```python
from build123d import *

# Parameters (mm, degrees)
F0_W     = 75.8
F0_H     = 10
F1_DEPTH = 2
F2_R     = 1
F4_D     = 3.5


with BuildPart() as f1:
    # F0 (on Front) → F1 (new body)
    with BuildSketch(Plane.XZ):
        Rectangle(F0_W, F0_H)
    extrude(amount=F1_DEPTH)

    # F2
    f2_edges = [f1.edges().sort_by_distance(p)[0] for p in [
        (-37.9, -1, 5),
        (37.9, -1, 5),
    ]]
    fillet(f2_edges, radius=F2_R)

    # F4 (through all)
    with Locations(Plane.XZ.offset(2)):
        with Locations((30, -0.5), (-30, -0.5)):
            Hole(F4_D / 2)


solid = f1.part
```
Verification items for the finished model (mm, model axes). Give positions to 0.01 mm unless a question says otherwise; leave off trailing zeros. Order: outer loops, then holes, each group sorted by start corner. A loop starts at its lowest first (then second) coordinate and runs counter-clockwise, first axis right, second up. Notation, with made-up numbers: M 16,-4 L 35,-4 A9 cw 35,1 Z; hole C 52.25,2 d8. An arc over 180 degrees is marked long. Answer in a Markdown table with one row per item. Add a question column.
Item 1: Section check B-B, the plane x = 30. Enter the section's corners in (y, z), and give its area (3 significant figures).
Item 2: Section check A-A, the plane z = -0.5. Enter the section's corners in (x, y), and give its area (3 significant figures).
Item 3: Scan lines: probe 1 along Z at (x, y) = (30, -0.85); probe 2 along X at (y, z) = (-0.9, 0.5); probe 3 along X at (y, z) = (-0.75, -1.75). Record each from-to range of solid material in increasing order. Write a range as from..to.
Item 4: Mould release check, pull along Z, two halves, no side actions. Record for faces 1 (the flat face through (-1, -1, -5)), 2 (the flat face through (-1, 0, 0)), 3 (the cylindrical face through (31.75, -0.99, -0.42)): released by +Z, released by -Z, zero draft, split by the parting line, or undercut.
Item 5: Section check C-C, the plane y = -1.3. Enter the section's corners in (x, z), and give its area (3 significant figures).
Filled sheet:
| question | item | result |
|---|---|---|
| 1 | outline | M -2,-5 L 0,-5 L 0,-2.25 L -2,-2.25 Z; M -2,1.25 L 0,1.25 L 0,5 L -2,5 Z |
| 1 | area | 13.0 mm^2 |
| 2 | outline | M -37.9,-2 L -31.75,-2 L -31.75,0 L -37.9,0 Z; M -28.25,-2 L 28.25,-2 L 28.25,0 L -28.25,0 Z; M 31.75,-2 L 37.9,-2 L 37.9,0 L 31.75,0 Z |
| 2 | area | 138 mm^2 |
| 3 | probe 1 | z = -5..-2.25, 1.25..5 |
| 3 | probe 2 | x = -37.9..-31.44, -28.56..28.56, 31.44..37.9 |
| 3 | probe 3 | x = -37.9..-31.22, -28.78..28.78, 31.22..37.9 |
| 4 | face 1 | released by -Z |
| 4 | face 2 | zero draft |
| 4 | face 3 | undercut |
| 5 | outline | M -37.9,-5 L 37.9,-5 L 37.9,4 A1 ccw 36.9,5 L -36.9,5 A1 ccw -37.9,4 Z; hole C -30,-0.5 d3.5; hole C 30,-0.5 d3.5 |
| 5 | area | 738 mm^2 |
